Work out the finished part from the listing and answer in its coordinate system (mm). Coordinates: 2 decimals unless noted, no trailing zeros. Loops run counter-clockwise (first coordinate to the right, second up) from the corner with the lowest first, then second, coordinate; pieces in that order, holes last. Notation, with made-up numbers: M 64,-17.75 L 91,-17.75 A11 ccw 91,-13.75 Z; hole C 73,89 d2. An arc over 180 degrees is marked long. Write each question's results on one line, items separated by ' | '.
```python
from build123d import *

# Parameters (mm, degrees)
BOSS_EXTRUDE1_DEPTH                     = 1.6
ENCLOSURE_MOUNTING_HOLES_M3_CLEARANCE_D = 3.4
BULKHEAD_MOUNTING_HOLES_M4X0_7_TAPPED_D = 3.3
SKETCH14_R                              = 1.7
CUT_EXTRUDE1_DEPTH                      = 82.171141516
CUT_EXTRUDE3_DEPTH                      = 10


with BuildPart() as part:
    # Sketch1 → Boss-Extrude1 (new body)
    with BuildSketch(Plane(origin=(0, 0, 0), x_dir=(1, 0, 0), z_dir=(0, 1, 0))):
        with BuildLine():
            Line((-48.093300583, -47.950176286), (-48.093300583, 47.950176286))
            ThreePointArc((-48.093300583, 47.950176286), (-47.660075225, 49.985997832), (-46.435472835, 51.669031572))
            ThreePointArc((-46.435472835, 51.669031572), (-36.474980605, 59.122903776), (-25.344708101, 64.680659646))
            ThreePointArc((-25.344708101, 64.680659646), (-18.640624701, 64.891621686), (-13.31129345, 60.818850193))
            ThreePointArc((-13.31129345, 60.818850193), (0, 53.594), (13.31129345, 60.818850193))
            ThreePointArc((13.31129345, 60.818850193), (18.640624701, 64.891621686), (25.344708101, 64.680659646))
            ThreePointArc((25.344708101, 64.680659646), (36.474980605, 59.122903776), (46.435472835, 51.669031572))
            ThreePointArc((46.435472835, 51.669031572), (47.660075225, 49.985997832), (48.093300583, 47.950176286))
            Line((48.093300583, 47.950176286), (48.093300583, -47.950176286))
            ThreePointArc((48.093300583, -47.950176286), (47.660075225, -49.985997832), (46.435472835, -51.669031572))
            ThreePointArc((46.435472835, -51.669031572), (36.474980605, -59.122903776), (25.344708101, -64.680659646))
            ThreePointArc((25.344708101, -64.680659646), (18.640624701, -64.891621686), (13.31129345, -60.818850193))
            ThreePointArc((13.31129345, -60.818850193), (0, -53.594), (-13.31129345, -60.818850193))
            ThreePointArc((-13.31129345, -60.818850193), (-18.640624701, -64.891621686), (-25.344708101, -64.680659646))
            ThreePointArc((-25.344708101, -64.680659646), (-36.474980605, -59.122903776), (-46.435472835, -51.669031572))
            ThreePointArc((-46.435472835, -51.669031572), (-47.660075225, -49.985997832), (-48.093300583, -47.950176286))
        make_face()
    extrude(amount=-BOSS_EXTRUDE1_DEPTH)

    # Enclosure Mounting Holes - M3 Clearance Hole1 (through all)
    with Locations(Plane(origin=(0, 0, 0), x_dir=(1, 0, 0), z_dir=(0, 1, 0))):
        with Locations((-36.8, 41.8), (-36.8, -41.8), (36.8, -41.8), (36.8, 41.8)):
            Hole(ENCLOSURE_MOUNTING_HOLES_M3_CLEARANCE_D / 2)

    # Bulkhead Mounting Holes - M4x0.7 Tapped Hole1 (through all)
    with Locations(Plane(origin=(0, 0, 0), x_dir=(1, 0, 0), z_dir=(0, 1, 0))):
        with Locations((-25, 55), (25, 55), (25, -55), (-25, -55)):
            Hole(BULKHEAD_MOUNTING_HOLES_M4X0_7_TAPPED_D / 2)

    # Sketch14 → Cut-Extrude1 (cut, through all)
    with BuildSketch(Plane(origin=(0, 0, 0), x_dir=(1, 0, 0), z_dir=(0, 1, 0))):
        with Locations(Location((42.75, -31.8, 0), (0, 0, 270))):
            Circle(SKETCH14_R)
    extrude(amount=-CUT_EXTRUDE1_DEPTH, mode=Mode.SUBTRACT)

    # Sketch17 → Cut-Extrude3 (cut)
    with BuildSketch(Plane(origin=(0, 0, 0), x_dir=(1, 0, 0), z_dir=(0, 1, 0))):
        Polygon((-26.8, -41.8), (-41.8, -26.8), (-41.8, 26.8), (-26.8, 41.8), (26.8, 41.8), (41.8, 26.8), (41.8, -26.8), (26.8, -41.8), align=None)
    extrude(amount=-CUT_EXTRUDE3_DEPTH, mode=Mode.SUBTRACT)


solid = part.part
```
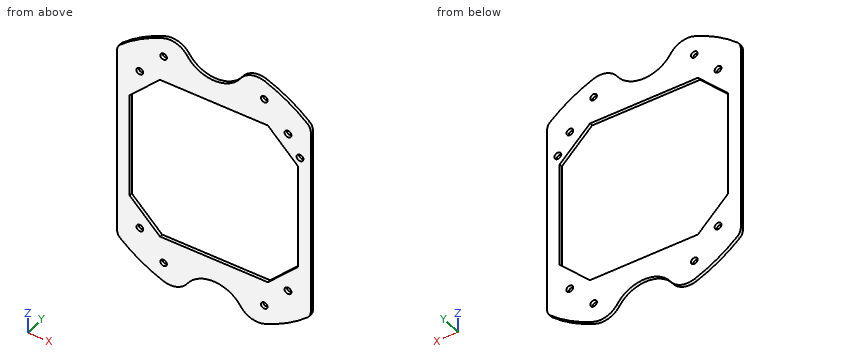
1) Find section C-C, the plane y = -1.15. Give the number of separate pieces and of enclosed holes in the cut face, and give its area (3 significant figures).
Check result:
separate pieces: 1 | enclosed holes: 10 | area: 4,760 mm^2
2) Given pin 1 Ø5.5 at (x, z) = (-36.8, 41.8) entering from +Y; pin 2 Ø0.5 at (x, y) = (7, -0.5) entering from +Z, each flat-ended and moving along its own axis, determine where each tip first touches the part or whether it passes through.
Check result:
pin 1: y = 0 | pin 2: z = 55.35
3) Find section B-B, the plane x = -5.5. Give the vertices of the cut face in (y, z).
Check result:
outline: M -1.6,-54.58 L 0,-54.58 L 0,-41.8 L -1.6,-41.8 Z; M -1.6,41.8 L 0,41.8 L 0,54.58 L -1.6,54.58 Z
4) Find section D-D, the plane z = 31.8. Give the vertices of the cut face in (x, y), and give its area (3 significant figures).
Check result:
outline: M -48.09,-1.6 L -36.8,-1.6 L -36.8,0 L -48.09,0 Z; M 36.8,-1.6 L 41.05,-1.6 L 41.05,0 L 36.8,0 Z; M 44.45,-1.6 L 48.09,-1.6 L 48.09,0 L 44.45,0 Z | area: 30.7 mm^2
5) Straight lines are drawn through the part: probe 1 along X at (y, z) = (-0.2, -22); probe 2 along X at (y, z) = (-1.2, 55); probe 3 along Z at (x, y) = (25, -0.5). For each, find the intervals that lie inside material, in ascending order. Write a range as [from, to].
Check result:
probe 1: [-48.09, -41.8], [41.8, 48.09] | probe 2: [-42.44, -26.65], [-23.35, -6.53], [6.53, 23.35], [26.65, 42.44] | probe 3: [-64.81, -56.65], [-53.35, -41.8], [41.8, 53.35], [56.65, 64.81]
6) Find section A-A, the plane z = 15.5. Give the vertices of the cut face in (x, y), and give its area (3 significant figures).
Check result:
outline: M -48.09,-1.6 L -41.8,-1.6 L -41.8,0 L -48.09,0 Z; M 41.8,-1.6 L 48.09,-1.6 L 48.09,0 L 41.8,0 Z | area: 20.1 mm^2
